Check sheet for the modelled part. Datum: model origin and axes. Units: mm. A direction names the side the tool comes from. Give positions to 0.01 mm unless a question says otherwise; leave off trailing zeros. Loops run counter-clockwise (first coordinate to the right, second up) from the corner with the lowest first, then second, coordinate; pieces in that order, holes last. Notation, with made-up numbers: M -28.5,11 L -2.5,11 A13 cw -2.5,18 Z; hole C -19.75,-13 d1. An arc over 180 degrees is marked long. Put each result on its own line as item: value. Start each with the question number.
Autodesk Inventor part; units mm, degrees
ref_plane "YZ Plane" through (0, 0, 0) normal (1, 0, 0) x (0, 1, 0)
ref_plane "XZ Plane" through (0, 0, 0) normal (0, 1, 0) x (-1, 0, 0)
ref_plane "XY Plane" through (0, 0, 0) normal (0, 0, 1) x (1, 0, 0)
sketch "Sketch1" plane through (0, 0, 0) normal (1, 0, 0) x (0, 1, 0)
  circle A0 centre (0, 0) radius 3.175
  dimension "d0" = 6.35
extrude "Extrusion1" add sketch "Sketch1" along normal blind 9.525
sketch "Sketch2" plane through (9.525, 0, 0) normal (1, 0, 0) x (0, 0, -1)
  circle A0 centre (0, 0) radius 5.3975
  dimension "d3" = 10.795
extrude "Extrusion2" add sketch "Sketch2" along normal blind 3.175
sketch "Sketch3" plane through (12.7, 0, 0) normal (1, 0, 0) x (0, 0, -1)
  line L0 (0, 0) -> (1.9812, 0)
  line L1 (0, 0) -> (-1.9812, 0)
  circle A0 centre (0, 0) radius 3.175
  line L2 (0, 0) -> (0.9906, 1.7158)
  line L3 (0, 0) -> (1.9812, 0) construction
  line L4 (0.9906, 1.7158) -> (1.9812, 0)
  line L5 (0, 0) -> (-0.9906, 1.7158)
  line L6 (0, 0) -> (1.9812, 0) construction
  line L7 (-0.9906, 1.7158) -> (0.9906, 1.7158)
  line L8 (-0.9906, 1.7158) -> (-1.9812, 0)
  line L9 (0, 0) -> (0.9906, -1.7158)
  line L10 (0, 0) -> (1.9812, 0) construction
  line L11 (0.9906, -1.7158) -> (1.9812, 0)
  line L12 (0, 0) -> (-0.9906, -1.7158)
  line L13 (0, 0) -> (1.9812, 0) construction
  line L14 (-0.9906, -1.7158) -> (0.9906, -1.7158)
  line L15 (-0.9906, -1.7158) -> (-1.9812, 0)
  dimension "d6" = 1.9812
  dimension "d7" = 1.9812
  dimension "d8" = 1.9812
  dimension "d9" = 60
  dimension "d10" = 1.9812
  dimension "d11" = 120
  dimension "d12" = 1.9812
  dimension "d13" = 60
  dimension "d14" = 1.9812
  dimension "d15" = 120
extrude "Extrusion3" cut sketch "Sketch3" against normal blind 3.175 contours L2 L4 L0 | L12 L15 L1 | L5 L7 L2 | L1 L8 L5 | L0 L11 L9 | L9 L14 L12
fillet "Fillet1" radius 3.175 1 edges at (12.7, 0, 5.3975)
thread "Thread1"
properties part number "1-4-20 screw"
Q1. Access from +Z, -Z, +X, -X, +Y, -Y to the whole of each face (thin tool, end or side, straight path). Record for faces 1 (the face through (12.7, 2, 0)), 2 (the face through (11.13, -0.87, 1.48)).
Q2. Mould release check, pull along Y, two halves, no side actions. Record for faces 3 (the face through (4.7, -0.69, 3.1)), 4 (the face through (9.525, -4, 0)), 5 (the face through (11.13, 0.87, -1.48)): pulls with the +Y half, pulls with the -Y half, needs draft (parallel to the pull), parting line crosses it, or undercut.
Q3. Section check A-A, the plane x = 6.5. Record the cut outline in (y, z) (3 decimals).
Q4. Depth check by flat-ended pin: P1, Ø1.5, axis at y = 0.5, z = 0.5, coming from the +X side (3 decimals); P2, Ø1.5, axis at x = 1.5, z = 1.5, coming from the -Y side; P3, Ø1, axis at x = 11, z = 0.5, coming from the +Y side. Enter the tip coordinate at first touch or a pass-through.
Q5. Thickness scan on line 1 along Z through (x, y) = (6, 0) (3 decimals); line 2 along Z through (x, y) = (11.25, -1); line 3 along X through (y, z) = (0.5, 0) (3 decimals). Record the ranges inside material, lowest first. Write a range as [from, to].
Found:
1. face 1: +Z, -Z, +X, +Y, -Y
1. face 2: +X
2. face 3: parting line crosses it
2. face 4: needs draft
2. face 5: undercut
3. outline: C 0,0 d6.35
4. P1: stops at x = 9.525
4. P2: stops at y = -3.09
4. P3: stops at y = 5.23
5. line 1: z = [-3.175, 3.175]
5. line 2: z = [-4.78, -1.4], [1.4, 4.78]
5. line 3: x = [0, 9.525]
